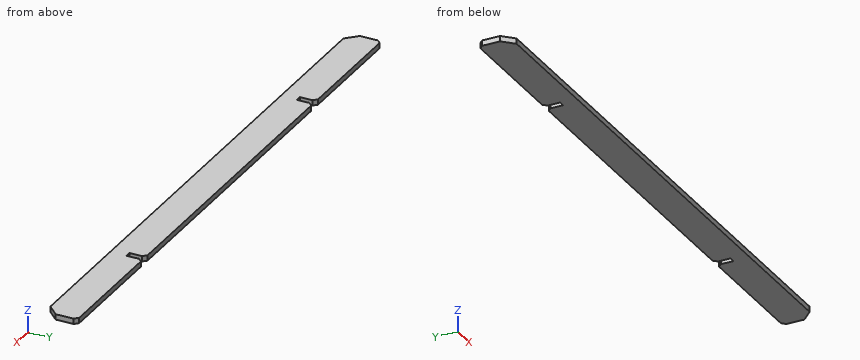
Autodesk Inventor part; units mm, degrees
ref_plane "YZ Plane" through (0, 0, 0) normal (1, 0, 0) x (0, 1, 0)
ref_plane "XZ Plane" through (0, 0, 0) normal (0, 1, 0) x (-1, 0, 0)
ref_plane "XY Plane" through (0, 0, 0) normal (0, 0, 1) x (1, 0, 0)
sketch "Sketch1" plane through (0, 0, 0) normal (0, 0, 1) x (1, 0, 0)
  line L0 (0, 0) -> (327, 0)
  line L1 (327, 0) -> (327, 18)
  line L2 (327, 18) -> (0, 18)
  line L3 (0, 18) -> (0, 0)
  line L4 (163.5, 18) -> (163.5, 0)
  line L5 (73.5, 18) -> (70.3, 18)
  line L6 (70.3, 18) -> (70.3, 9)
  line L7 (70.3, 9) -> (73.5, 9)
  line L8 (73.5, 9) -> (73.5, 18)
  line L9 (256.7, 18) -> (256.7, 9)
  line L10 (256.7, 9) -> (253.5, 9)
  line L11 (253.5, 9) -> (253.5, 18)
  dimension "d0" = 327
  dimension "d1" = 18
  dimension "d2" = 3.2
  dimension "d3" = 9
  dimension "d4" = 180
extrude "Plate1" add sketch "Sketch1" along normal blind 3 contours L3 L2 L6 L7 L8 L4 L0 | L4 L2 L11 L10 L9 L1 L0
chamfer "Corner Chamfer1" distance 6 angle 45 2 edges at (0, 0, 1.5) (327, 0, 1.5)
chamfer "Corner Chamfer2" distance 2 angle 45 6 edges at (327, 18, 1.5) (256.7, 18, 1.5) (253.5, 18, 1.5) (73.5, 18, 1.5) (70.3, 18, 1.5) (0, 18, 1.5)
equation "\"d5\" = Thickness"
equation "\"BendRadius\" = Thickness"
equation "\"BendReliefWidth\" = Thickness"
equation "\"BendReliefDepth\" = 0.5 * Thickness"
equation "\"CornerReliefSize\" = 4 * Thickness"
equation "\"MinimumRemnant\" = 2 * Thickness"
equation "\"TransitionRadius\" = BendRadius"
equation "\"JacobiRadiusSize\" = BendRadius"
equation "\"GapSize\" = Thickness"
properties part number "foot support"
Model file for the job. Use its own axes, mm. Give positions to 0.01 mm unless a question says otherwise; leave off trailing zeros. Loops run counter-clockwise (first coordinate to the right, second up) from the corner with the lowest first, then second, coordinate; pieces in that order, holes last. Notation, with made-up numbers: (21.5, 16.25) - (47.5, 16.25) arc R6 cw to (47.5, 26.25) - close; hole circle Ø4 at (49, 16). An arc over 180 degrees is marked (long way). One line per item, written item: value. Start each with the question number.
1. Pin check, flat tips, straight feed: pin 1 (0.9 mm diameter, centred on x = 255.5, z = 1.5, fed in from +Y); pin 2 (1.5 mm diameter, centred on y = 2.5, z = 1.5, fed in from -X); pin 3 (0.9 mm diameter, centred on y = 13, z = 1, fed in from -X). Stop position of each tip, or through.
2. Probe L1, parallel to X at y = 10.25, z = 1.5; L2, parallel to X at y = 5.75, z = 0.9; L3, parallel to X at y = 4.25, z = 2.9. List the from-to ranges inside material, lowest first. Write a range as from..to.
3. Slice it at A-A (y = 12.25). List the corners of the cut face in (x, z).
4. Slice it at B-B (z = 1.95). List the corners of the cut face in (x, y).
Solution:
1. pin 1: stops at y = 9
1. pin 2: stops at x = 2.75
1. pin 3: stops at x = 0
2. L1: x = 0..70.3, 73.5..253.5, 256.7..327
2. L2: x = 0.25..326.75
2. L3: x = 1.75..325.25
3. outline: (0, 0) - (70.3, 0) - (70.3, 3) - (0, 3) - close; (73.5, 0) - (253.5, 0) - (253.5, 3) - (73.5, 3) - close; (256.7, 0) - (327, 0) - (327, 3) - (256.7, 3) - close
4. outline: (0, 6) - (6, 0) - (321, 0) - (327, 6) - (327, 16) - (325, 18) - (258.7, 18) - (256.7, 16) - (256.7, 9) - (253.5, 9) - (253.5, 16) - (251.5, 18) - (75.5, 18) - (73.5, 16) - (73.5, 9) - (70.3, 9) - (70.3, 16) - (68.3, 18) - (2, 18) - (0, 16) - close
